Autodesk Inventor part; units mm, degrees
ref_plane "YZ Plane" through (0, 0, 0) normal (1, 0, 0) x (0, 1, 0)
ref_plane "XZ Plane" through (0, 0, 0) normal (0, 1, 0) x (-1, 0, 0)
ref_plane "XY Plane" through (0, 0, 0) normal (0, 0, 1) x (1, 0, 0)
sketch "Sketch1" plane through (0, 0, 0) normal (0, 1, 0) x (-1, 0, 0)
  circle A0 centre (0, 0) radius 73.025
  line L0 (0, 0) -> (0, -73.025) construction
  line L1 (0, 0) -> (-12.6807, -71.9156)
  line L2 (0, 0) -> (12.6807, -71.9156)
  line L3 (0, 0) -> (72.3143, -10.1631)
  line L4 (0, 0) -> (64.4772, -34.2832)
  line L5 (0, 0) -> (32.0121, 65.6344)
  line L6 (0, 0) -> (52.5298, 50.7274)
  line L7 (0, 0) -> (-52.5298, 50.7274)
  line L8 (0, 0) -> (-32.0121, 65.6344)
  line L9 (0, 0) -> (-64.4772, -34.2832)
  line L10 (0, 0) -> (-72.3143, -10.1631)
  circle A1 centre (0, 0) radius 69.85
  arc A2 (4.7597, -69.6876) -> (-4.7597, -69.6876) centre (0, -69.85) ccw
  arc A3 (67.7477, -17.0079) -> (64.806, -26.0614) centre (66.4313, -21.5848) ccw
  arc A4 (37.1107, 59.1762) -> (44.8121, 53.5808) centre (41.0568, 56.5098) ccw
  arc A5 (-44.8121, 53.5808) -> (-37.1107, 59.1762) centre (-41.0568, 56.5098) ccw
  arc A6 (-64.806, -26.0614) -> (-67.7477, -17.0079) centre (-66.4313, -21.5848) ccw
  point P0 (61.6739, -32.7926)
  point P1 (69.1702, -9.7212)
  point P2 (50.2459, 48.5219)
  point P3 (30.6202, 62.7808)
  point P4 (-30.6202, 62.7808)
  point P5 (-50.2459, 48.5219)
  point P6 (-69.1702, -9.7212)
  point P7 (-61.6739, -32.7926)
  point P8 (-12.1293, -68.7888)
  point P9 (12.1293, -68.7888)
  point P10 (64.806, -26.0614)
  point P11 (67.7477, -17.0079)
  point P12 (44.8121, 53.5808)
  point P13 (37.1107, 59.1762)
  point P14 (-37.1107, 59.1762)
  point P15 (-67.7477, -17.0079)
  dimension "d0" = 146.05
  dimension "d1" = 10
  dimension "d4" = 360
  dimension "d6" = 3.175
  dimension "d10" = 9.525
  dimension "d13" = 360
extrude "Extrusion1" add sketch "Sketch1" along normal blind 6.35 contours A0 L3 A1 L6 | L5 A1 L8 A0 | A1 L3 L6 | L6 L5 A1 A4 | A0 L2 A1 L4 | A1 A3 L4 L3 | L5 L8 A1 | L2 A1 A2 L1 | L4 A1 L2 | L10 A1 L7 | L7 A1 A5 L8 | L1 A1 L9 | L9 A1 A6 L10 | L7 A1 L10 A0 | L1 A0 L9 A1
fillet "Fillet1" radius 1.5875 30 edges at (30.6202, 3.175, 62.7808) (32.0121, 3.175, 65.6344) (-30.6202, 3.175, 62.7808) (-32.0121, 3.175, 65.6344) (-52.5298, 3.175, 50.7274) (-50.2459, 3.175, 48.5219) (52.5298, 3.175, 50.7274) (50.2459, 3.175, 48.5219) (64.4772, 3.175, -34.2832) (61.6739, 3.175, -32.7926) (72.3143, 3.175, -10.1631) (69.1702, 3.175, -9.7212) (12.6807, 3.175, -71.9156) (12.1293, 3.175, -68.7888) (-12.6807, 3.175, -71.9156) (-12.1293, 3.175, -68.7888) (-72.3143, 3.175, -10.1631) (-69.1702, 3.175, -9.7212) (-64.4772, 3.175, -34.2832) (-61.6739, 3.175, -32.7926) (37.1107, 3.175, 59.1762) (44.8121, 3.175, 53.5808) (-44.8121, 3.175, 53.5808) (-37.1107, 3.175, 59.1762) (-64.806, 3.175, -26.0614) (-67.7477, 3.175, -17.0079) (4.7597, 3.175, -69.6876) (-4.7597, 3.175, -69.6876) (67.7477, 3.175, -17.0079) (64.806, 3.175, -26.0614)
sketch "Sketch5" plane through (0, 6.35, 0) normal (0, 1, 0) x (1, 0, 0)
  line L0 (0, 0) -> (0, 65.0875) construction
  arc A0 (-4.554, 68.4564) -> (4.554, 68.4564) centre (0, 69.85) ccw
  circle A1 centre (0, 50.8) radius 22.225 construction
  arc A2 (63.6995, 35.7075) -> (14.2757, 71.616) centre (0, 0) ccw
  circle A3 centre (-24.6062, 60.325) radius 1.7526
  circle A4 centre (-24.6062, 60.325) radius 3.175
  circle A5 centre (-22.225, 34.925) radius 3.175
  circle A6 centre (-22.225, 34.925) radius 1.7526
  circle A7 centre (24.6062, 60.325) radius 1.7526
  circle A8 centre (24.6062, 60.325) radius 3.175
  circle A9 centre (22.225, 34.925) radius 3.175
  circle A10 centre (22.225, 34.925) radius 1.7526
  arc A11 (6.2133, 69.5731) -> (4.554, 68.4564) centre (6.0721, 67.9919) ccw
  arc A12 (6.2133, 69.5731) -> (4.554, 68.4564) centre (6.0721, 67.9919) ccw
  arc A13 (-4.554, 68.4564) -> (-6.2133, 69.5731) centre (-6.0721, 67.9919) ccw
  arc A14 (-4.554, 68.4564) -> (-6.2133, 69.5731) centre (-6.0721, 67.9919) ccw
  arc A15 (-12.4019, 70.3348) -> (-10.5977, 69.0414) centre (-10.8385, 70.6105) ccw
  arc A16 (10.5977, 69.0414) -> (12.4019, 70.3348) centre (10.8385, 70.6105) ccw
  arc A17 (10.5977, 69.0414) -> (6.2133, 69.5731) centre (0, 0) ccw
  arc A18 (10.5977, 69.0414) -> (11.9875, 69.515) centre (10.8385, 70.6105) ccw
  arc A19 (-6.2133, 69.5731) -> (-10.5977, 69.0414) centre (0, 0) ccw
  arc A20 (-14.2757, 71.616) -> (-63.6995, 35.7075) centre (0, 0) ccw
  line L1 (-28.4451, 67.2572) -> (-25.3861, 34.6286) construction
  line L2 (-22.7046, 31.7864) -> (-3.3572, 28.83) construction
  line L3 (28.4451, 67.2572) -> (25.3861, 34.6286) construction
  line L4 (22.7046, 31.7864) -> (3.3572, 28.83) construction
  circle A21 centre (0, 0) radius 73.025
  circle A22 centre (0, 50.8) radius 19.05 construction
  arc A23 (-27.365, 61.8966) -> (-24.6436, 32.868) centre (-5.295, 49.3238) ccw
  arc A24 (-21.8475, 58.7534) -> (-19.8064, 36.982) centre (-5.295, 49.3238) ccw
  point P0 (-63.6995, 35.7075)
  point P1 (-9.2869, 69.2299)
  point P2 (9.2869, 69.2299)
  point P3 (-5.0165, 69.1776)
  point P4 (5.0165, 69.1776)
  point P5 (14.2757, 71.616)
  dimension "d40" = 44.45
  dimension "d41" = 3.5052
  dimension "d42" = 6.35
  dimension "d43" = 9.525
  dimension "d44" = 24.6062
  dimension "d45" = 6.35
  dimension "d46" = 3.5052
  dimension "d47" = 15.875
  dimension "d48" = 22.225
  dimension "d70" = 38.1
  dimension "d72" = 25.4
  dimension "d73" = 19.05
extrude "Extrusion3" cut sketch "Sketch5" against normal blind 25.4 contours A21 A20 A2 | A3 | A6 | A7 | A8 | A9 | A10
equation "\"d45\" = d42"
equation "\"d46\" = d41"
properties part number "Top Plate" material "Nylon 6/6"
CAD build for the part. Positions are in the model's coordinates, mm. Give positions to 0.01 mm unless a question says otherwise; leave off trailing zeros. Order: outer loops, then holes, each group sorted by start corner. A loop starts at its lowest first (then second) coordinate and runs counter-clockwise, first axis right, second up.
(1) Saw through at D-D, the plane x = -29.75. Give the cut face in (y, z).
(2) Mould opens along X. For faces 1 (the cylindrical face through (-24.276, 3.219, -47.708)), 2 (the cylindrical face through (-20.222, 3.219, -32.462)), 3 (the flat face through (-26, 0, -47)), 4 (the cylindrical face through (-23.8, 3.22, -58.77)) say: released by +X, released by -X, zero draft, split by the parting line, or undercut.
(3) Saw through at B-B, the plane y = 0.5. State how many separate pieces and enclosed holes the cut face has, then the cut area to 3 significant figures.
(4) Flat gauge pins, fed straight in: pin 1 (3 mm diameter, centred on x = -25, y = 4.5, fed in from +Z); pin 2 (2 mm diameter, centred on y = 1.5, z = -57.5, fed in from -X); pin 3 (2 mm diameter, centred on y = 3, z = -45.5, fed in from +X); pin 4 (3 mm diameter, centred on x = -21, z = -51.5, fed in from -Y). Where does each tip first touch, or does it go through?
(5) Saw through at C-C, the plane z = -51. Give the cut face in (x, y), then the cut area to 3 significant figures.
(6) Drill centre lines: L1, parallel to Z at x = -22, y = 2.5; L2, parallel to X at y = 0.75, z = -35.5; L3, parallel to Z at x = -22.5, y = 3. Where is each one in solid material? Low to high.
(7) Saw through at A-A, the plane x = -26. Give the cut face in (y, z), then the cut area to 3 significant figures.
Results found:
1. outline: (0, -56.19) - (6.35, -56.19) - (6.35, -42.46) - (0, -42.46) - close
2. face 1: released by +X
2. face 2: split by the parting line
2. face 3: zero draft
2. face 4: undercut
3. separate pieces: 1
3. enclosed holes: 2
3. area: 185 mm2
4. pin 1: stops at z = -32.02
4. pin 2: stops at x = -29.66
4. pin 3: stops at x = -23.72
4. pin 4: passes through
5. outline: (-30.64, 0) - (-24.27, 0) - (-24.27, 6.35) - (-30.64, 6.35) - close
5. area: 40.4 mm2
6. L1: z = -62.14 to -58.48, -40.17 to -36.66, -33.19 to -31.76
6. L2: x = -26.6 to -23.88, -20.57 to -19.1
6. L3: z = -62.7 to -57.5, -41.15 to -36.66, -33.19 to -31.76
7. outline: (0, -63.18) - (6.35, -63.18) - (6.35, -61.39) - (0, -61.39) - close; (0, -59.26) - (6.35, -59.26) - (6.35, -34.61) - (0, -34.61) - close
7. area: 168 mm2
